```python
from build123d import *

# Parameters (mm, degrees)
SKETCH1_W           = 41
SKETCH1_H           = 20
BOSS_EXTRUDE1_DEPTH = 6
NUT_DEPTH           = 4
SKETCH7_R           = 2.75
HOLES_DEPTH         = 7


with BuildPart() as part:
    # Sketch1 → Boss-Extrude1 (new body)
    with BuildSketch(Plane(origin=(0, 0, 0), x_dir=(1, 0, 0), z_dir=(0, 1, 0))):
        with Locations((20.5, 10)):
            Rectangle(SKETCH1_W, SKETCH1_H)
    extrude(amount=-BOSS_EXTRUDE1_DEPTH)

    # Sketch2 → nut (cut)
    with BuildSketch(Plane(origin=(0, 0, 0), x_dir=(1, 0, 0), z_dir=(0, 1, 0))):
        Polygon((20.5, 5.150257739), (24.7, 7.575128869), (24.7, 12.424871131), (20.5, 14.849742261), (16.3, 12.424871131), (16.3, 7.575128869), align=None)
    extrude(amount=-NUT_DEPTH, mode=Mode.SUBTRACT)

    # Sketch7 → holes (cut, through all)
    with BuildSketch(Plane(origin=(0, 0, 0), x_dir=(1, 0, 0), z_dir=(0, 1, 0))):
        with Locations((8.5, 10)):
            Circle(SKETCH7_R)
        with Locations((32.5, 10)):
            Circle(SKETCH7_R)
        with Locations((20.5, 10)):
            Circle(SKETCH7_R)
    extrude(amount=-HOLES_DEPTH, mode=Mode.SUBTRACT)


solid = part.part
```
Input: part model. Units: mm. Frame: model coordinates. A direction names the side the tool comes from. Give positions to 0.01 mm unless a question says otherwise; leave off trailing zeros. Order: outer loops, then holes, each group sorted by start corner. A loop starts at its lowest first (then second) coordinate and runs counter-clockwise, first axis right, second up. Notation, with made-up numbers: (88, 69) - (99, 69) arc R29 cw to (99, 92) - close; hole circle Ø9 at (-5, 78). An arc over 180 degrees is marked (long way). Put each result on its own line as item: value.
Item 1: Section query C-C, the plane z = -8. Return loops of the section in (x, y), then the cut area to 3 significant figures.
Found:
outline: (0, -6) - (6.61, -6) - (6.61, 0) - (0, 0) - close; (10.39, -6) - (18.61, -6) - (18.61, -4) - (16.3, -4) - (16.3, 0) - (10.39, 0) - close; (22.39, -6) - (30.61, -6) - (30.61, 0) - (24.7, 0) - (24.7, -4) - (22.39, -4) - close; (34.39, -6) - (41, -6) - (41, 0) - (34.39, 0) - close
area: 160 mm^2
Item 2: Section query A-A, the plane x = 32.5. Return loops of the section in (y, z), then the cut area to 3 significant figures.
Found:
outline: (-6, -20) - (0, -20) - (0, -12.75) - (-6, -12.75) - close; (-6, -7.25) - (0, -7.25) - (0, 0) - (-6, 0) - close
area: 87.0 mm^2
Item 3: Access query for faces 1 (the cylindrical face through (8.142, -2.958, -12.727)), 2 (the flat face through (24.7, -2, -10)). Directions: +Z, -Z, +X, -X, +Y, -Y. A direction counts if a zero-diameter tool reaches every point of the face in a straight line with its end or side. Return the directions, or none.
Found:
face 1: +Y, -Y
face 2: +Y
Item 4: Draft query along X for faces 3 (the flat face through (41, -3, -10)), 4 (the flat face through (0, -3, -10)), 5 (the flat face through (16, -6, -10)), 6 (the flat face through (16.3, -2, -10)). Return one class per face: +X half, -X half, draft (parallel to the pull), parting line (faces both ways), or undercut.
Found:
face 3: +X half
face 4: -X half
face 5: draft
face 6: undercut
Item 5: Contact query for a flat-ended pin moving along its axis: pin 1 (4 mm diameter, centred on x = 19, z = -8.5, fed in from +Y). Output: stop coordinate, or through.
Found:
pin 1: stops at y = -4
Item 6: Section query D-D, the plane y = -1.4. Return loops of the section in (x, z).
Found:
outline: (0, -20) - (41, -20) - (41, 0) - (0, 0) - close; hole circle Ø5.5 at (8.5, -10); hole (16.3, -12.42) - (20.5, -14.85) - (24.7, -12.42) - (24.7, -7.58) - (20.5, -5.15) - (16.3, -7.58) - close; hole circle Ø5.5 at (32.5, -10)
Item 7: Section query B-B, the plane y = -5.3. Return loops of the section in (x, z), then the cut area to 3 significant figures.
Found:
outline: (0, -20) - (41, -20) - (41, 0) - (0, 0) - close; hole circle Ø5.5 at (8.5, -10); hole circle Ø5.5 at (20.5, -10); hole circle Ø5.5 at (32.5, -10)
area: 749 mm^2
Item 8: Ray query, L1, parallel to X at y = -2.2, z = -10; L2, parallel to X at y = -5.1, z = -10; L3, parallel to Z at x = 32.5, y = -2.8. Return the intervals inside material, ascending. Write a range as from..to.
Found:
L1: x = 0..5.75, 11.25..16.3, 24.7..29.75, 35.25..41
L2: x = 0..5.75, 11.25..17.75, 23.25..29.75, 35.25..41
L3: z = -20..-12.75, -7.25..0
